Drawing for the job (mm, zero at the part's lowest x, y, z). Coordinates: 2 decimals unless noted, no trailing zeros. Write each loop counter-clockwise with the first axis right and the second up, starting at its lowest first coordinate (ties: lowest second). Pieces come first, ordered by that corner, then holes. Notation, with made-up numbers: (-37.75, 58) - (2.25, 58) arc R12 cw to (2.25, 75) - close; hole circle Ø11 at (13, 62). An arc over 180 degrees is marked (long way). Write each question's results on one line, items separated by ' | '.
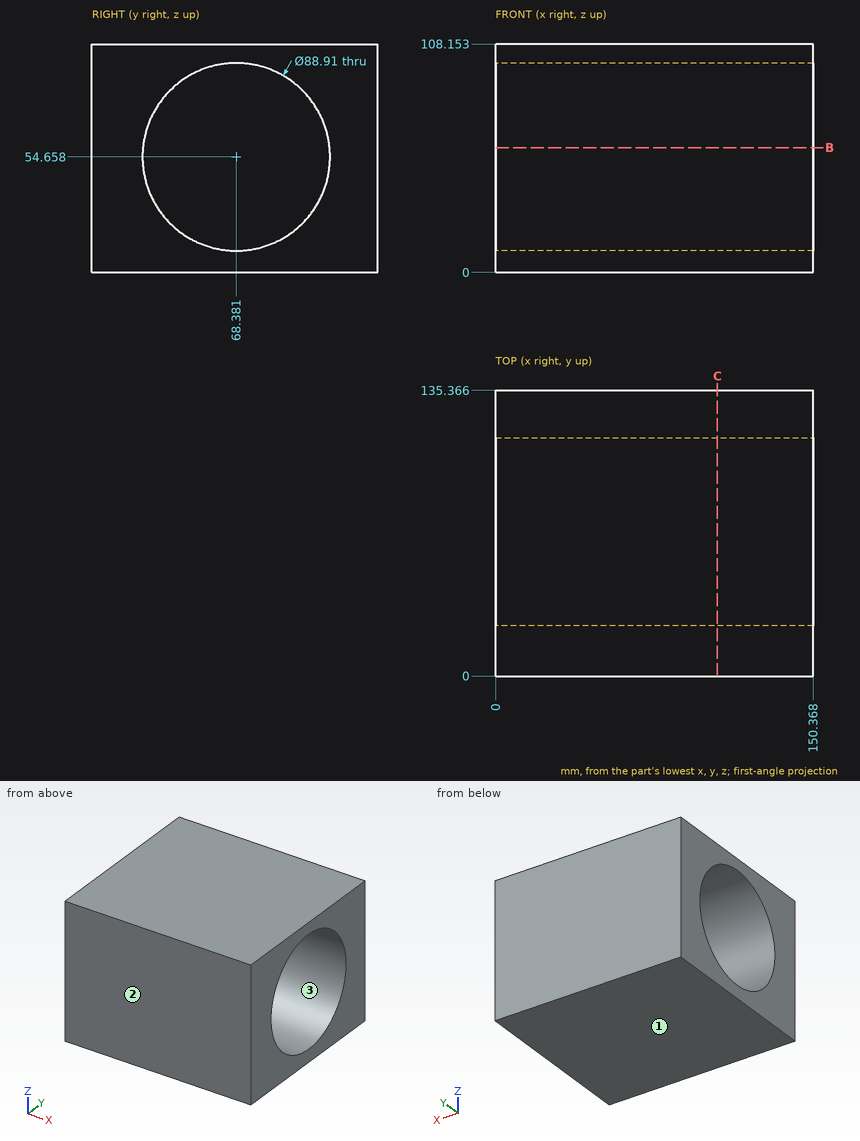
(1) Wall check: line 1 (Z direction, x = 56, y = 100.5) (1 decimal); line 2 (Y direction, x = 103.5, z = 77) (1 decimal); line 3 (Y direction, x = 53, z = 57) (1 decimal). Give the ranges that are in metal, low to high. Write a range as from..to.
Return value:
line 1: z = 0..23.9, 85.4..108.2 | line 2: y = 0..29.9, 106.8..135.4 | line 3: y = 0..24, 112.8..135.4
(2) Saw through at C-C on x = 105. Write the cut outline in (y, z) (1 decimal), then the cut area to 3 significant figures.
Return value:
outline: (0, 0) - (135.4, 0) - (135.4, 108.2) - (0, 108.2) - close; hole circle Ø88.9 at (68.4, 54.7) | area: 8,430 mm^2
(3) Saw through at B-B on z = 59. Write the cut outline in (x, y) (1 decimal), then the cut area to 3 significant figures.
Return value:
outline: (0, 0) - (150.4, 0) - (150.4, 24.1) - (0, 24.1) - close; (0, 112.6) - (150.4, 112.6) - (150.4, 135.4) - (0, 135.4) - close | area: 7,050 mm^2
(4) Two-plate mould, pull along Y, no slides. Class the marked faces 1, 2 and 3: released by +Y, released by -Y, zero draft, split by the parting line, or undercut.
Return value:
face 1: zero draft | face 2: released by -Y | face 3: undercut
